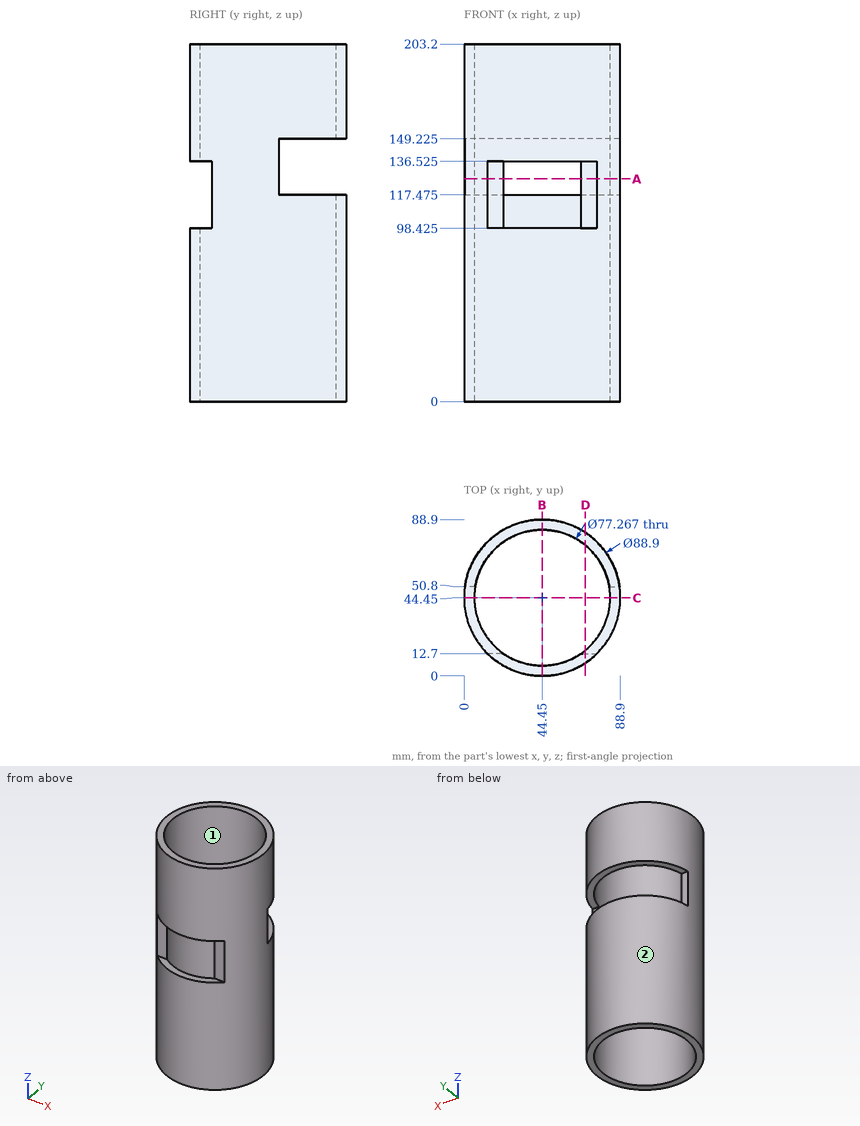
Verification items for this drawing (mm, ordinates from the low corner). Coordinates: 2 decimals unless noted, no trailing zeros. Order: outer loops, then holes, each group sorted by start corner. A loop starts at its lowest first (then second) coordinate and runs counter-clockwise, first axis right, second up. Notation, with made-up numbers: M 65.25,-0.75 L 101.25,-0.75 A20 ccw 101.25,19.25 Z; hole C -3.75,53 d10. An arc over 180 degrees is marked long. Use CSV: the item, a comma, the result in double quotes.
Item 1: Gauge pin test, flat ends, axial feed: pin 1 Ø3 at (x, z) = (66.5, 66) entering from +Y (1 decimal); pin 2 Ø5 at (x, z) = (28, 47) entering from -Y; pin 3 Ø2.5 at (x, z) = (70, 111) entering from -Y; pin 4 Ø19 at (x, y) = (57, 69) entering from +Z. Record the tip position at first contact, or that the pin passes through.
Returned:
pin 1,"stops at y = 83.9"
pin 2,"stops at y = 2.25"
pin 3,"stops at y = 12.7"
pin 4,"passes through"
Item 2: Thickness scan on line 1 along X through (y, z) = (44, 87); line 2 along Y through (x, z) = (51, 110) (1 decimal); line 3 along Y through (x, z) = (39, 86) (1 decimal). Record the ranges inside material, lowest first.
Returned:
line 1,"x = 0 to 5.82, 83.08 to 88.9"
line 2,"y = 82.5 to 88.4"
line 3,"y = 0.3 to 6.2, 82.7 to 88.6"
Item 3: Cross-section at B-B on x = 44.45. Record the cut outline in (y, z) (1 decimal), then the cut area to 3 significant figures.
Returned:
outline,"M 0,0 L 5.8,0 L 5.8,98.4 L 0,98.4 Z; M 0,136.5 L 5.8,136.5 L 5.8,203.2 L 0,203.2 Z; M 83.1,0 L 88.9,0 L 88.9,117.5 L 83.1,117.5 Z; M 83.1,149.2 L 88.9,149.2 L 88.9,203.2 L 83.1,203.2 Z"
area,"1,960 mm2"
Item 4: Mould release check, pull along Y, two halves, no side actions. Record for the marked faces 1 and 2: pulls with the +Y half, pulls with the -Y half, needs draft (parallel to the pull), parting line crosses it, or undercut.
Returned:
face 1,"undercut"
face 2,"parting line crosses it"
Item 5: Cross-section at D-D on x = 69. Record the cut outline in (y, z) (1 decimal).
Returned:
outline,"M 7.4,0 L 14.6,0 L 14.6,203.2 L 7.4,203.2 L 7.4,136.5 L 12.7,136.5 L 12.7,98.4 L 7.4,98.4 Z; M 74.3,0 L 81.5,0 L 81.5,117.5 L 74.3,117.5 Z; M 74.3,149.2 L 81.5,149.2 L 81.5,203.2 L 74.3,203.2 Z"
Item 6: Cross-section at C-C on y = 44.45. Record the cut outline in (x, z), then the cut area to 3 significant figures.
Returned:
outline,"M 0,0 L 5.82,0 L 5.82,203.2 L 0,203.2 Z; M 83.08,0 L 88.9,0 L 88.9,203.2 L 83.08,203.2 Z"
area,"2,360 mm2"
Item 7: Cross-section at A-A on z = 126.5. Record the cut outline in (x, y), then the cut area to 3 significant figures.
Returned:
outline,"M 0.46,50.8 A44.45 ccw 13.34,12.7 L 22.44,12.7 A38.63 cw 6.34,50.8 Z; M 66.46,12.7 L 75.56,12.7 A44.45 ccw 88.44,50.8 L 82.56,50.8 A38.63 cw Z"
area,"495 mm2"
